from build123d import *
from OCP.BRepFilletAPI import BRepFilletAPI_MakeChamfer

# Parameters (mm, degrees)
CROQUIS1_W                 = 140
CROQUIS1_H                 = 45
SALIENTE_EXTRUIR1_DEPTH    = 40
CORTAR_EXTRUIR1_DEPTH      = 84.703345214
CORTAR_EXTRUIR1_DEPTH_BACK = 84.703345214
CROQUIS2_W                 = 74
CROQUIS2_H                 = 42
CROQUIS3_R                 = 6.55
CORTAR_EXTRUIR2_DEPTH      = 80
CROQUIS10_R                = 8.55
CROQUIS10_R_2              = 6.55
SALIENTE_EXTRUIR3_DEPTH    = 3.35
CORTAR_EXTRUIR3_REACH      = 92.907
CROQUIS4_R                 = 1.651
CROQUIS5_R                 = 4.5
CROQUIS5_R_2               = 3.5
SALIENTE_EXTRUIR2_DEPTH    = 3
CHAFL_N3_SIZE              = 3
CORTAR_EXTRUIR5_DEPTH      = 84.703345214
CORTAR_EXTRUIR5_DEPTH_BACK = 84.703345214
REDONDEO1_R                = 4
CHAFL_N1_SIZE              = 10
CHAFL_N1_SIZE2             = 5
CHAFL_N2_SIZE              = 5
CHAFL_N2_SIZE2             = 10


with BuildPart() as part:
    # Croquis1 → Saliente-Extruir1 (new, symmetric)
    with BuildSketch(Plane.XY):
        Rectangle(CROQUIS1_W, CROQUIS1_H)
    extrude(amount=SALIENTE_EXTRUIR1_DEPTH, both=True)

    # Croquis2 → Cortar-Extruir1 (cut, two sides: drawn at the far end of the back side and taken through both)
    with BuildSketch(Plane(origin=(0, 0, 0), x_dir=(0, 0, -1), z_dir=(1, 0, 0)).offset(-CORTAR_EXTRUIR1_DEPTH_BACK)):
        with Locations((0, -1.5)):
            Rectangle(CROQUIS2_W, CROQUIS2_H)
    extrude(amount=CORTAR_EXTRUIR1_DEPTH + CORTAR_EXTRUIR1_DEPTH_BACK, mode=Mode.SUBTRACT)

    # Croquis3 → Cortar-Extruir2 (cut)
    with BuildSketch(Plane.XY.offset(40)):
        with Locations((50, -10)):
            Circle(CROQUIS3_R)
        with Locations((-50, -10)):
            Circle(CROQUIS3_R)
    extrude(amount=-CORTAR_EXTRUIR2_DEPTH, mode=Mode.SUBTRACT)

    # Croquis10 → Saliente-Extruir3 (add)
    # profile 1 of 2: a face of its own
    with BuildSketch(Plane(origin=(0, 0, 37), x_dir=(-1, 0, 0), z_dir=(0, 0, -1))):
        with Locations(Location((-50, -10, 0), (0, 0, 270))):
            Circle(CROQUIS10_R)
        with Locations(Location((-50, -10, 0), (0, 0, 180))):
            Circle(CROQUIS10_R_2, mode=Mode.SUBTRACT)
    # profile 2 of 2: a face of its own
    with BuildSketch(Plane(origin=(0, 0, 37), x_dir=(-1, 0, 0), z_dir=(0, 0, -1))):
        with Locations(Location((50, -10, 0), (0, 0, 270))):
            Circle(CROQUIS10_R)
        with Locations(Location((50, -10, 0), (0, 0, 180))):
            Circle(CROQUIS10_R_2, mode=Mode.SUBTRACT)
    saliente_extruir3 = extrude(amount=SALIENTE_EXTRUIR3_DEPTH)

    # Simetría1: Saliente-Extruir3 across plane
    add(saliente_extruir3.mirror(Plane.XY))

    # Croquis4 → Cortar-Extruir3 (cut, up to next)
    with BuildSketch(Plane.XZ.offset(-19.5), mode=Mode.PRIVATE) as cortar_extruir3_sk1:
        with Locations(Location((-65, 25, 0), (0, 0, 270))):
            Circle(CROQUIS4_R)
    cortar_extruir3_tool1 = extrude(cortar_extruir3_sk1.sketch, amount=-CORTAR_EXTRUIR3_REACH, mode=Mode.PRIVATE) & part.part
    # Croquis4 → Cortar-Extruir3 (cut, up to next)
    with BuildSketch(Plane.XZ.offset(-19.5), mode=Mode.PRIVATE) as cortar_extruir3_sk2:
        with Locations(Location((-65, -25, 0), (0, 0, 270))):
            Circle(CROQUIS4_R)
    cortar_extruir3_tool2 = extrude(cortar_extruir3_sk2.sketch, amount=-CORTAR_EXTRUIR3_REACH, mode=Mode.PRIVATE) & part.part
    cortar_extruir3_1 = cortar_extruir3_tool1.solids().sort_by_distance((-65, 19.5, 25))[0]
    add(cortar_extruir3_1, mode=Mode.SUBTRACT)
    cortar_extruir3_2 = cortar_extruir3_tool2.solids().sort_by_distance((-65, 19.5, -25))[0]
    add(cortar_extruir3_2, mode=Mode.SUBTRACT)
    cortar_extruir3 = cortar_extruir3_1 + cortar_extruir3_2  # Cortar-Extruir3 as one shape, for the pattern or mirror that repeats it

    # Croquis5 → Saliente-Extruir2 (add)
    # profile 1 of 2: a face of its own
    with BuildSketch(Plane.XZ.offset(-19.5)):
        with Locations(Location((-65, 25, 0), (0, 0, 90))):
            Circle(CROQUIS5_R)
        with Locations(Location((-65, 25, 0), (0, 0, 270))):
            Circle(CROQUIS5_R_2, mode=Mode.SUBTRACT)
    # profile 2 of 2: a face of its own
    with BuildSketch(Plane.XZ.offset(-19.5)):
        with Locations(Location((-65, -25, 0), (0, 0, 90))):
            Circle(CROQUIS5_R)
        with Locations(Location((-65, -25, 0), (0, 0, 270))):
            Circle(CROQUIS5_R_2, mode=Mode.SUBTRACT)
    saliente_extruir2 = extrude(amount=SALIENTE_EXTRUIR2_DEPTH)

    # Simetría2: Cortar-Extruir3, Saliente-Extruir2 across plane
    add(cortar_extruir3.mirror(Plane(origin=(0, 0, 0), x_dir=(0, 0, 1), z_dir=(1, 0, 0))), mode=Mode.SUBTRACT)
    add(saliente_extruir2.mirror(Plane(origin=(0, 0, 0), x_dir=(0, 0, 1), z_dir=(1, 0, 0))))

    # Chaflán3
    chafl_n3_edges = [part.edges().sort_by_distance(p)[0] for p in [
        (50, -1.45, 37),
        (-50, -1.45, 37),
        (50, -1.45, -37),
        (-50, -1.45, -37),
    ]]
    chamfer(chafl_n3_edges, length=CHAFL_N3_SIZE)

    # Croquis9 → Cortar-Extruir5 (cut, two sides: drawn at the far end of the back side and taken through both)
    with BuildSketch(Plane.XY.offset(-CORTAR_EXTRUIR5_DEPTH_BACK)):
        Polygon((-40, -22.5), (-35, 19.5), (35, 19.5), (40, -22.5), align=None)
        Polygon((-70, 7.5), (-60, -22.5), (-70, -22.5), align=None)
        Polygon((70, 7.5), (60, -22.5), (70, -22.5), align=None)
    extrude(amount=CORTAR_EXTRUIR5_DEPTH + CORTAR_EXTRUIR5_DEPTH_BACK, mode=Mode.SUBTRACT)

    # Redondeo1
    redondeo1_edges = [part.edges().sort_by_distance(p)[0] for p in [
        (40, -22.5, 38.5),
        (40, -22.5, -38.5),
        (-35, 19.5, 38.5),
        (-35, 19.5, -38.5),
        (-40, -22.5, -38.5),
        (-40, -22.5, 38.5),
        (35, 19.5, -38.5),
        (35, 19.5, 38.5),
        (-70, 7.5, 38.5),
        (-70, 7.5, -38.5),
        (-60, -22.5, 38.5),
        (-60, -22.5, -38.5),
        (70, 7.5, 38.5),
        (70, 7.5, -38.5),
        (60, -22.5, 38.5),
        (60, -22.5, -38.5),
    ]]
    fillet(redondeo1_edges, radius=REDONDEO1_R)

    # Chaflán1: one chamfer whose edges measure the first distance from different faces: ONE call of the kernel's chamfer builder (chamfer() names one face for all edges)
    chafl_n1_edges_1 = [part.edges().sort_by_distance(p)[0] for p in [
        (50.723972764, 19.5, -37),
    ]]
    chafl_n1_side_1 = [part.faces().sort_by_distance(p)[0] for p in [
        (53.195449018, 6.150722288, -37),
    ]]
    chafl_n1_edges_2 = [part.edges().sort_by_distance(p)[0] for p in [
        (-50.723972764, 19.5, -37),
    ]]
    chafl_n1_side_2 = [part.faces().sort_by_distance(p)[0] for p in [
        (-53.195449018, 6.150722288, -37),
    ]]
    chafl_n1 = BRepFilletAPI_MakeChamfer(part.part.solid().wrapped)
    for e in chafl_n1_edges_1:
        chafl_n1.Add(CHAFL_N1_SIZE, CHAFL_N1_SIZE2, e.wrapped, chafl_n1_side_1[0].wrapped)  # the first distance lies on this face
    for e in chafl_n1_edges_2:
        chafl_n1.Add(CHAFL_N1_SIZE, CHAFL_N1_SIZE2, e.wrapped, chafl_n1_side_2[0].wrapped)  # the first distance lies on this face
    add(Compound.cast(chafl_n1.Shape()), mode=Mode.REPLACE)

    # Chaflán2
    chafl_n2_edges = [part.edges().sort_by_distance(p)[0] for p in [
        (50.723972764, 19.5, 37),
        (-50.723972764, 19.5, 37),
    ]]
    chafl_n2_side = [part.faces().sort_by_distance(p)[0] for p in [
        (0, 19.5, 1.317218046),
    ]]
    chamfer(chafl_n2_edges, length=CHAFL_N2_SIZE, length2=CHAFL_N2_SIZE2, reference=chafl_n2_side[0])


solid = part.part
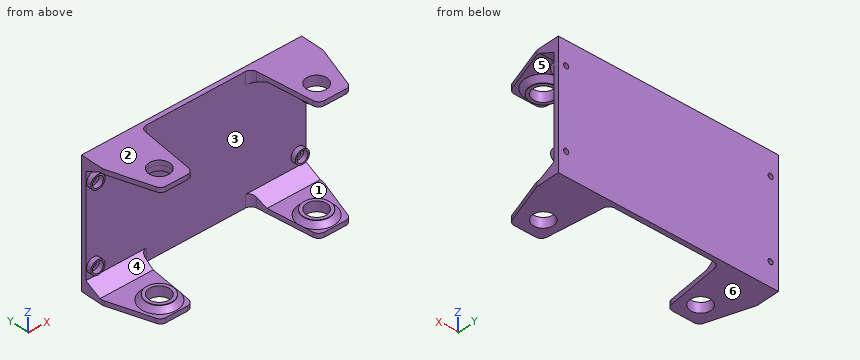
Model file for the job. Use its own axes, mm. Face numbers are marked on the shaded views. A direction names the side the tool comes from. Give positions to 0.01 mm unless a question says otherwise; leave off trailing zeros. Order: outer loops, then holes, each group sorted by start corner. A loop starts at its lowest first (then second) coordinate and runs counter-clockwise, first axis right, second up. Notation, with made-up numbers: M -19.5,24.5 L 21.5,24.5 A26 cw 21.5,49.5 Z; hole C 33.25,59 d3. An arc over 180 degrees is marked long. Put each result on its own line as item: value. Start each with the question number.
(1) Tool access for the marked faces 4, 5 and 6: list every direction of +Z, -Z, +X, -X, +Y, -Y with a clear straight run to the whole face (end or side of a thin tool).
(2) Band-saw the part on C-C on y = 11. Give the cut face in (x, z), then the cut area to 3 significant figures.
(3) Pin check, flat tips, straight feed: pin 1 Ø7 at (x, z) = (63.5, -25) entering from -Y; pin 2 Ø10 at (y, z) = (-8.5, 30) entering from +X; pin 3 Ø5 at (x, z) = (-34.5, -5.5) entering from -Y. Stop position of each tip, or through.
(4) Band-saw the part on A-A on x = 65. Count the separate pieces of the cut face and the enclosed holes in it, then the cut area to 3 significant figures.
(5) Band-saw the part on B-B on z = 25. Give the cut face in (x, y), then the cut area to 3 significant figures.
(6) Pull direction X, two halves, no side cores. Call the marked faces 1, 2 and 3: released by +X, released by -X, zero draft, split by the parting line, or undercut.
(7) Drill centre lines: L1, parallel to X at y = 17.7, z = -25; L2, parallel to X at y = 21, z = 25; L3, parallel to Y at x = 50, z = -37.5. Where is each one in solid material? Low to high. Write a range as [from, to].
Results below:
1. face 4: +X, -X
1. face 5: none
1. face 6: -Z, +X, -X, +Y, -Y
2. outline: M -70,-40 L -36.01,-40 L -36.01,-36.25 L -70,-36.25 Z; M -70,36.25 L -36.01,36.25 L -36.01,40 L -70,40 Z; M 36.01,-40 L 70,-40 L 70,-36.25 L 36.01,-36.25 Z; M 36.01,36.25 L 70,36.25 L 70,40 L 36.01,40 Z
2. area: 510 mm2
3. pin 1: stops at y = 16.5
3. pin 2: stops at x = 59.47
3. pin 3: stops at y = 19.5
4. separate pieces: 3
4. enclosed holes: 0
4. area: 444 mm2
5. outline: M -70,19.5 L -69.5,19.5 L -69.5,16.5 L -68.5,16.5 L -68.5,19.5 L -66.65,19.5 L -66.65,22.5 L -70,22.5 Z; M -63.35,19.5 L -61.5,19.5 L -61.5,16.5 L -60.5,16.5 L -60.5,19.5 L 60.5,19.5 L 60.5,16.5 L 61.5,16.5 L 61.5,19.5 L 63.35,19.5 L 63.35,22.5 L -63.35,22.5 Z; M 66.65,19.5 L 68.5,19.5 L 68.5,16.5 L 69.5,16.5 L 69.5,19.5 L 70,19.5 L 70,22.5 L 66.65,22.5 Z
5. area: 412 mm2
6. face 1: undercut
6. face 2: zero draft
6. face 3: undercut
7. L1: x = [-69.5, -68.5], [-61.5, -60.5], [60.5, 61.5], [68.5, 69.5]
7. L2: x = [-70, -66.65], [-63.35, 63.35], [66.65, 70]
7. L3: y = [-22.5, -16.55], [-3.45, 22.5]
